from build123d import *

# Parameters (mm, degrees)
F0_R         = 46.5
F0_R_2       = 45
F1_DEPTH     = 9
F3_DEPTH     = 25
F5_DEPTH     = 25
F7_DEPTH     = 9
F9_DEPTH     = 9
F11_DEPTH    = 9
F13_DEPTH    = 25
F15_DEPTH    = 25
F16_R        = 45
F17_DEPTH    = 9
F18_R        = 45
F19_DEPTH    = 25
F21_DEPTH    = 25
F22_R        = 1.55
F23_T1_DEPTH = 16.2900218994
F24_T1_DEPTH = 16.2900218994


# Not quite as in the source:
# - a fillet or chamfer that OpenCascade refuses, or shapes differently, is made with other operations: its cross-section is extruded or revolved along the edge and cut away or added


with BuildPart() as f1:
    # F0 (on Top) → F1 (new body)
    with BuildSketch(Plane.XY):
        Circle(F0_R)
        Circle(F0_R_2, mode=Mode.SUBTRACT)
    extrude(amount=F1_DEPTH)

    # F2 (on face) → F3 (cut)
    with BuildSketch(Plane.XY.offset(9)):
        Polygon((64.8135244846, -21.5104352683), (0, -21.5104352683), (-51.5724048018, -21.5104352683), (-51.5724048018, -59.9158406258), (64.033716917, -57.7713772655), align=None)
    extrude(amount=-F3_DEPTH, mode=Mode.SUBTRACT)

    # F4 (on face) → F5 (cut)
    with BuildSketch(Plane.XY.offset(9)):
        with BuildLine():
            ThreePointArc((-40.5525222975, -19.506228116), (-40.9032938672, -20.5072072896), (-41.9042730407, -20.1564357199))
            Line((-41.9042730407, -20.1564357199), (-43.4346050024, -22.7221362293))
            Line((-43.4346050024, -22.7221362293), (-36.3525599241, -23.4547629952))
            Line((-36.3525599241, -23.4547629952), (-40.5525222975, -19.506228116))
        make_face()
        with BuildLine():
            Line((43.4346050024, -22.7221362293), (41.9042730407, -20.1564357199))
            ThreePointArc((41.9042730407, -20.1564357199), (40.9032938672, -20.5072072896), (40.5525222975, -19.506228116))
            Line((40.5525222975, -19.506228116), (36.3525599241, -23.4547629952))
            Line((36.3525599241, -23.4547629952), (43.4346050024, -22.7221362293))
        make_face()
    extrude(amount=-F5_DEPTH, mode=Mode.SUBTRACT)

    # F6 (on face) → F7 (join)
    with BuildSketch(Plane.XY.offset(9)):
        with BuildLine():
            ThreePointArc((6.9320949163, 52.5), (-4.9017313232, 57.4017313232), (0, 45.5679050837))
            ThreePointArc((0, 45.5679050837), (4.9017313232, 47.5982686768), (6.9320949163, 52.5))
        make_face()
        with BuildLine():
            ThreePointArc((5, 52.5), (3.5355339059, 48.9644660941), (0, 47.5))
            ThreePointArc((0, 47.5), (-3.5355339059, 56.0355339059), (5, 52.5))
        make_face(mode=Mode.SUBTRACT)
    extrude(amount=-F7_DEPTH)

    # F8 (on face) → F9 (join)
    with BuildSketch(Plane.XY.offset(9)):
        with BuildLine():
            ThreePointArc((-6.9320949163, 52.5), (-7.6007884485, 48.9142518774), (-9.1181185374, 45.5972577502))
            ThreePointArc((-9.1181185374, 45.5972577502), (0, 45.60976302), (9.1181185374, 45.5972577502))
            ThreePointArc((9.1181185374, 45.5972577502), (7.6007884485, 48.9142518774), (6.9320949163, 52.5))
            ThreePointArc((6.9320949163, 52.5), (0, 47.0015761941), (-6.9320949163, 52.5))
        make_face()
    extrude(amount=-F9_DEPTH)

    # F10 (on face) → F11 (join)
    with BuildSketch(Plane.XY.offset(9)):
        with BuildLine():
            Line((-44.8310511788, 3.895747708), (-46.3451584316, 3.7916078319))
            ThreePointArc((-46.3451584316, 3.7916078319), (-42.7926175487, -9.5215818837), (-33.8443815708, -19.9996847659))
            ThreePointArc((-33.8443815708, -19.9996847659), (-32.8631083129, -20.2138563114), (-32.1503467858, -19.506228116))
            ThreePointArc((-32.1503467858, -19.506228116), (-41.2777702931, -9.315455738), (-44.8310511788, 3.895747708))
        make_face()
        with BuildLine():
            ThreePointArc((33.8443815708, -19.9996847659), (42.7926175487, -9.5215818837), (46.3451584316, 3.7916078319))
            Line((46.3451584316, 3.7916078319), (44.8310511788, 3.895747708))
            ThreePointArc((44.8310511788, 3.895747708), (41.2777702931, -9.315455738), (32.1503467858, -19.506228116))
            ThreePointArc((32.1503467858, -19.506228116), (32.8631083129, -20.2138563114), (33.8443815708, -19.9996847659))
        make_face()
    extrude(amount=-F11_DEPTH)

    # F12 (on face) → F13 (cut)
    with BuildSketch(Plane.XY.offset(9)):
        with BuildLine():
            ThreePointArc((-44.7172397739, -5.0367119241), (-45.830770977, -0.896267065), (-46.3787269492, 3.35614162))
            Line((-46.3787269492, 3.35614162), (-53.9689548314, -20.3920416534))
            Line((-53.9689548314, -20.3920416534), (-39.6306179464, -26.7084874213))
            Line((-39.6306179464, -26.7084874213), (-35.9670780599, -21.9711512327))
            Line((-35.9670780599, -21.9711512327), (-43.2941578329, -10.1593965665))
            Line((-43.2941578329, -10.1593965665), (-44.7172397739, -5.0367119241))
        make_face()
        with BuildLine():
            Line((53.9689548314, -20.3920416534), (46.3787269492, 3.35614162))
            ThreePointArc((46.3787269492, 3.35614162), (45.830770977, -0.896267065), (44.7172397739, -5.0367119241))
            Line((44.7172397739, -5.0367119241), (43.2941578329, -10.1593965665))
            Line((43.2941578329, -10.1593965665), (35.9670780599, -21.9711512327))
            Line((35.9670780599, -21.9711512327), (39.6306179464, -26.7084874213))
            Line((39.6306179464, -26.7084874213), (53.9689548314, -20.3920416534))
        make_face()
    extrude(amount=-F13_DEPTH, mode=Mode.SUBTRACT)

    # F14 (on face) → F15 (cut)
    with BuildSketch(Plane.XY.offset(9)):
        with BuildLine():
            ThreePointArc((-45.7581778434, -1.2523031469), (-46.1397679432, 3.2286956321), (-45.8552008738, 7.7169004675))
            ThreePointArc((-45.8552008738, 7.7169004675), (-48.5264373147, 3.20287819), (-45.7581778434, -1.2523031469))
        make_face()
        with BuildLine():
            ThreePointArc((45.7581778434, -1.2523031469), (48.5264373147, 3.20287819), (45.8552008738, 7.7169004675))
            ThreePointArc((45.8552008738, 7.7169004675), (46.1397679432, 3.2286956321), (45.7581778434, -1.2523031469))
        make_face()
    extrude(amount=-F15_DEPTH, mode=Mode.SUBTRACT)

    # F16 (on face) → F17 (join)
    with BuildSketch(Plane.XY.offset(9)):
        with BuildLine():
            ThreePointArc((-9.1181185374, 45.5972577502), (0, -46.5), (9.1181185374, 45.5972577502))
            ThreePointArc((9.1181185374, 45.5972577502), (0, 46.5), (-9.1181185374, 45.5972577502))
        make_face()
        Circle(F16_R, mode=Mode.SUBTRACT)
    extrude(amount=-F17_DEPTH)

    # F18 (on face) → F19 (cut)
    with BuildSketch(Plane.XY.offset(9)):
        Circle(F18_R)
    extrude(amount=-F19_DEPTH, mode=Mode.SUBTRACT)

    # F20 (on face) → F21 (cut)
    with BuildSketch(Plane.XY.offset(9)):
        Polygon((18, 0), (0, 0), (-18, 0), (-18, -69.9843019247), (18, -69.3941116333), align=None)
    extrude(amount=-F21_DEPTH, mode=Mode.SUBTRACT)

    # F22
    f22_edges = [f1.edges().sort_by_distance(p)[0] for p in [
        (-18, -41.243181, 4.5),
        (18, -41.243181, 4.5),
    ]]
    fillet(f22_edges, radius=F22_R)

    # F23: fillet of radius 1.5 on 1 edges, made by hand

    # F23_s2 → F23_t1 (cut)
    with BuildSketch(Plane.XY.offset(-3.6450109497)):
        with BuildLine():
            ThreePointArc((18, -42.2457098414), (18.6625262969, -42.4244445619), (19.3353236307, -42.2894225557))
            ThreePointArc((19.3353236307, -42.2894225557), (18.6699563348, -42.5873541143), (18, -42.8748177839))
            Line((18, -42.8748177839), (18, -42.2457098414))
        make_face()
    extrude(amount=F23_T1_DEPTH, mode=Mode.SUBTRACT)

    # F24: fillet of radius 1.5 on 1 edges, made by hand

    # F24_s2 → F24_t1 (cut)
    with BuildSketch(Plane.XY.offset(-3.6450109497)):
        with BuildLine():
            ThreePointArc((-18, -42.2457098414), (-18.6625262969, -42.4244445619), (-19.3353236307, -42.2894225557))
            ThreePointArc((-19.3353236307, -42.2894225557), (-18.6699563348, -42.5873541143), (-18, -42.8748177839))
            Line((-18, -42.8748177839), (-18, -42.2457098414))
        make_face()
    extrude(amount=F24_T1_DEPTH, mode=Mode.SUBTRACT)


solid = f1.part
Build history of the part. All positions in model axes, mm. Coordinates: 2 decimals unless noted, no trailing zeros. Order: outer loops, then holes, each group sorted by start corner. A loop starts at its lowest first (then second) coordinate and runs counter-clockwise, first axis right, second up. Notation, with made-up numbers: (-2.75, -16.75) - (26.25, -16.75) arc R19 cw to (26.25, 11.25) - close; hole circle Ø4 at (10, 18). An arc over 180 degrees is marked (long way). Put each result on its own line as item: value.
1. Probe line 1 along Y through (x, z) = (0, 3); line 2 along X through (y, z) = (0, 5.5); line 3 along X through (y, z) = (52.5, 5.5). List the from-to ranges inside material, lowest first. Write a range as [from, to].
Answer sheet:
line 1: y = [45, 47.5], [57.5, 59.43]
line 2: x = [-46.5, -45], [45, 46.5]
line 3: x = [-6.93, -5], [5, 6.93]
2. Pull direction X, two halves, no side cores. Call faces 1 (the face through (7.616, 48.865, 4.563)), 2 (the face through (-17, 43, 0)), 3 (the face through (0.15, 59.43, 4.56)), 4 (the face through (1.706, 44.968, 4.563)): pulls with the +X half, pulls with the -X half, needs draft (parallel to the pull), parting line crosses it, or undercut.
Answer sheet:
face 1: pulls with the +X half
face 2: needs draft
face 3: parting line crosses it
face 4: undercut
3. Saw through at D-D (x = 14). Write the cut outline in (y, z), and give its area (3 significant figures).
Answer sheet:
outline: (42.77, 0) - (44.34, 0) - (44.34, 9) - (42.77, 9) - close
area: 14.2 mm^2
4. Saw through at B-B (y = 0). Write the cut outline in (x, z), and give its area (3 significant figures).
Answer sheet:
outline: (-46.5, 0) - (-45, 0) - (-45, 9) - (-46.5, 9) - close; (45, 0) - (46.5, 0) - (46.5, 9) - (45, 9) - close
area: 27.0 mm^2
5. Saw through at A-A (z = 4.5). Write the cut outline in (x, y), and give its area (3 significant figures).
Answer sheet:
outline: (-19.34, -42.29) arc R1.5 ccw to (-18, -42.25) arc R1.55 ccw to (-18.9, -40.84) arc R45 cw (long way) to (18.9, -40.84) arc R1.55 ccw to (18, -42.25) arc R1.5 ccw to (19.34, -42.29) arc R46.5 ccw to (9.12, 45.6) arc R14.95 cw to (6.93, 52.5) arc R6.93 ccw to (-6.93, 52.5) arc R14.95 cw to (-9.12, 45.6) arc R46.5 ccw to start; hole circle Ø10 at (0, 52.5)
area: 467 mm^2
6. Drop flat-ended pins along their axis: P1, Ø1, axis at y = 41, z = 4.5, coming from the -X side; P2, Ø3, axis at x = -13, z = 4, coming from the -Y side. Give the stop position or say it passes through.
Answer sheet:
P1: stops at x = -22.85
P2: stops at y = 42.6
7. Saw through at C-C (x = -23.5). Write the cut outline in (y, z).
Answer sheet:
outline: (-40.12, 0) - (-38.38, 0) - (-38.38, 9) - (-40.12, 9) - close; (38.38, 0) - (40.12, 0) - (40.12, 9) - (38.38, 9) - close
